Input: part model. Units: mm. Frame: model coordinates. Face numbers are marked on the shaded views. A direction names the side the tool comes from. Round coordinates to 2 decimals unless told otherwise and drop trailing zeros. Loops run counter-clockwise (first coordinate to the right, second up) from the corner with the lowest first, then second, coordinate; pieces in that order, holes last. Notation, with made-up numbers: M -32,51 L 25,51 A29 ccw 25,82 Z; hole C -35,-3.5 d8. An arc over 180 degrees is marked long. Put each result on its own line as item: value. Start each with the question number.
1) Section D-D on z = 34. Output: boundary loops of the cut face in (x, y), plus the area to 3 significant figures.
2) Reachability of the marked faces 5, 6, 7 and 8 from +Z, -Z, +X, -X, +Y, -Y: full face, straight path, thin tool, end or side. Return the list, or none.
3) Pin query (flat end, axial travel): pin 1 (1.5 mm diameter, centred on x = -10.5, z = 20, fed in from -Y); pin 2 (5 mm diameter, centred on x = -14.5, z = 31, fed in from +Y); pin 3 (3 mm diameter, centred on y = -9, z = 21.5, fed in from -X). Return the tip coordinate at first contact, or that it passes through.
4) Line query: probe 1 along Z at (x, y) = (10.5, -6.5); probe 2 along Y at (x, z) = (-26.5, 7); probe 3 along X at (y, z) = (24, 3). Output: solid intervals per line, ascending.
5) Section C-C on x = -23. Output: boundary loops of the cut face in (y, z), plus the area to 3 significant figures.
6) Draft query along Z for the marked faces 1, 2, 3 and 4. Return one class per face: +Z half, -Z half, draft (parallel to the pull), parting line (faces both ways), or undercut.
7) Section B-B on x = -9.5. Output: boundary loops of the cut face in (y, z).
8) Section A-A on z = 6. Output: boundary loops of the cut face in (x, y).
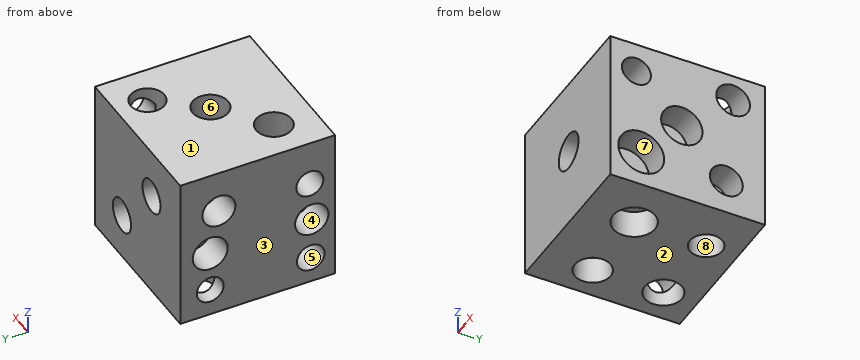
from build123d import *

# Parameters (mm, degrees)
F0_W      = 45.548788
F0_H      = 43.902439
F1_DEPTH  = 44
F3_R      = 5.278003
F4_DEPTH  = 6.1
F6_R      = 4.792021
F6_R_2    = 4.833087
F7_DEPTH  = 8.7
F9_R      = 5.007153
F9_R_2    = 5.037139
F9_R_3    = 4.799872
F10_DEPTH = 9.9
F11_R     = 5.299354
F11_R_2   = 5.083632
F11_R_3   = 4.607541
F11_R_4   = 5.974621
F12_DEPTH = 7.9
F14_R     = 4.115857
F14_R_2   = 4.79202
F14_R_3   = 5.865796
F14_R_4   = 6.522182
F14_R_5   = 4.672699
F15_DEPTH = 8.3
F17_R     = 3.928671
F17_R_2   = 4.73671
F17_R_3   = 3.851249
F17_R_4   = 3.81195
F17_R_5   = 4.969419
F17_R_6   = 4.688783
F18_DEPTH = 9


with BuildPart() as f1:
    # F0 (on Top) → F1 (new body)
    with BuildSketch(Plane.XY):
        with Locations((-8.368903, 7.542874)):
            Rectangle(F0_W, F0_H)
    extrude(amount=F1_DEPTH)

    # F3 (on offset) → F4 (cut)
    with BuildSketch(Plane.XZ.offset(14.9)):
        with Locations((-7.820123, 22.634339)):
            Circle(F3_R)
    extrude(amount=-F4_DEPTH, mode=Mode.SUBTRACT)

    # F6 (on offset) → F7 (cut)
    with BuildSketch(Plane.XZ.offset(-30.2)):
        with Locations((-15.777439, 30.042876)):
            Circle(F6_R)
        with Locations((0, 13.03068)):
            Circle(F6_R_2)
    extrude(amount=F7_DEPTH, mode=Mode.SUBTRACT)

    # F9 (on offset) → F10 (cut)
    with BuildSketch(Plane.XY.offset(45.6)):
        with Locations((-20.164827, -2.881098)):
            Circle(F9_R)
        with Locations((-6.445313, 7.82012)):
            Circle(F9_R_2)
        with Locations((3.432736, 20.442074)):
            Circle(F9_R_3)
    extrude(amount=-F10_DEPTH, mode=Mode.SUBTRACT)

    # F11 (on Top) → F12 (cut)
    with BuildSketch(Plane.XY):
        with Locations((-21.811167, 19.893292)):
            Circle(F11_R)
        with Locations((-22.085557, 0)):
            Circle(F11_R_2)
        with Locations((0, 20.442074)):
            Circle(F11_R_3)
        Circle(F11_R_4)
    extrude(amount=F12_DEPTH, mode=Mode.SUBTRACT)

    # F14 (on offset) → F15 (cut)
    with BuildSketch(Plane.YZ.offset(14.6)):
        with Locations((-6.996952, 35.530679)):
            Circle(F14_R)
        with Locations((20.442074, 36.353853)):
            Circle(F14_R_2)
        with Locations((5.89939, 22.90873)):
            Circle(F14_R_3)
        with Locations((-5.625001, 10.286777)):
            Circle(F14_R_4)
        with Locations((18.521342, 10.012387)):
            Circle(F14_R_5)
    extrude(amount=-F15_DEPTH, mode=Mode.SUBTRACT)

    # F17 (on offset) → F18 (cut)
    with BuildSketch(Plane.YZ.offset(-31.3)):
        with Locations((-7.545732, 7.54859)):
            Circle(F17_R)
        with Locations((-7.820123, 19.621762)):
            Circle(F17_R_2)
        with Locations((-7.271341, 31.146152)):
            Circle(F17_R_3)
        with Locations((20.990856, 7.82298)):
            Circle(F17_R_4)
        with Locations((20.990856, 19.34737)):
            Circle(F17_R_5)
        with Locations((18.521342, 31.969324)):
            Circle(F17_R_6)
    extrude(amount=F18_DEPTH, mode=Mode.SUBTRACT)


solid = f1.part
Geometry results:
1. outline: M -31.14,-14.41 L 14.41,-14.41 L 14.41,-10.82 L 6.3,-10.82 L 6.3,-3.18 L 14.41,-3.18 L 14.41,16.27 L 6.3,16.27 L 6.3,24.62 L 14.41,24.62 L 14.41,29.49 L -13.07,29.49 L -13.07,21.5 L -18.48,21.5 L -18.48,29.49 L -31.14,29.49 L -31.14,22.75 L -22.3,22.75 L -22.3,14.3 L -31.14,14.3 L -31.14,-4.69 L -22.3,-4.69 L -22.3,-9.86 L -31.14,-9.86 Z
1. area: 1,710 mm²
2. face 5: -X
2. face 6: +Z
2. face 7: +X
2. face 8: -Z
3. pin 1: stops at y = -8.8
3. pin 2: stops at y = 21.5
3. pin 3: stops at x = -22.3
4. probe 1: z = 0 to 3.82, 16.75 to 31.44, 39.62 to 44
4. probe 2: y = -14.41 to -11.44, -3.66 to -2.52, 2.52 to 17.27, 24.71 to 29.49
4. probe 3: x = -31.14 to -25.16, -18.46 to -2.93, 2.93 to 14.41
5. outline: M -14.41,0 L -5,0 L -5,4.56 A3.93 cw long -3.63,7.9 L 5,7.9 L 5,0 L 14.73,0 L 14.73,7.9 L 17.18,7.9 A3.81 cw 24.8,7.9 L 25.06,7.9 L 25.06,0 L 29.49,0 L 29.49,44 L 1.25,44 L 1.25,35.7 L -7.01,35.7 L -7.01,44 L -14.41,44 Z; hole C -7.82,19.62 d9.47; hole C -7.27,31.15 d7.7; hole C 18.52,31.97 d9.38; hole C 20.99,19.35 d9.94
5. area: 1,370 mm²
6. face 1: +Z half
6. face 2: -Z half
6. face 3: draft
6. face 4: undercut
7. outline: M -14.41,0 L 29.49,0 L 29.49,44 L 11.83,44 L 11.83,35.7 L 3.81,35.7 L 3.81,44 L -14.41,44 L -14.41,27.64 L -8.8,27.64 L -8.8,17.63 L -14.41,17.63 Z
8. outline: M -31.14,-14.41 L 14.41,-14.41 L 14.41,-10.54 L 6.3,-10.54 L 6.3,-0.71 L 14.41,-0.71 L 14.41,16.13 L 6.3,16.13 L 6.3,20.92 L 14.41,20.92 L 14.41,29.49 L -31.14,29.49 L -31.14,24.34 L -24.7,24.34 A5.3 cw long -26.61,17.64 L -31.14,17.64 L -31.14,-3.94 L -25.3,-3.94 A5.08 cw long -22.3,-5.08 L -22.3,-11.16 L -31.14,-11.16 Z; hole C 0,0 d11.95; hole C 0,20.44 d9.22
